For this review, take the finished solid that the model builds, in its own axes (mm). Face numbers are marked on the shaded views. A direction names the side the tool comes from. Coordinates: 2 decimals unless noted, no trailing zeros. Loops run counter-clockwise (first coordinate to the right, second up) from the corner with the lowest first, then second, coordinate; pieces in that order, holes last. Notation, with made-up numbers: (44.25, 62) - (54.25, 62) arc R29 cw to (54.25, 95) - close; hole circle Ø5 at (-20.5, 19.25). An arc over 180 degrees is marked (long way). Answer as a JSON object with one key per item and string values. Group by question number.
Item 1: We need section A-A (z = 11). Give the boundary of the cut face in (x, y).
Item 2: Tool access review of the marked faces 4 and 5: name each direction out of +Z, -Z, +X, -X, +Y, -Y from which nothing blocks a thin tool from reaching the whole face with its end or side.
Item 3: Mouldability with a two-part tool opening along X and no side actions: class the marked faces 1, 2 and 3 as released by +X, released by -X, zero draft, split by the parting line, or undercut.
Item 4: We need section C-C (z = 18). Give the boundary of the cut face in (x, y).
Item 5: To check wall thickness, follow line 1 (X direction, y = -19.1, z = 25); line 2 (Z direction, x = 7.5, y = -18); line 3 (Z direction, x = 8, y = -18.8). State the ranges of each line that lie inside material, in increasing order.
Item 6: We need section D-D (y = 3). Give the boundary of the cut face in (x, z).
Item 7: We need section B-B (x = 0). Give the boundary of the cut face in (y, z), then the cut area to 3 significant figures.
Item 8: Clearance check with flat-ended pins moving along their axes: pin 1 (10 mm diameter, centred on x = 3, y = -15, fed in from +Z); pin 2 (13 mm diameter, centred on x = 0, z = 18, fed in from +Y); pin 3 (2 mm diameter, centred on x = 2, y = 9, fed in from +Z). State where each tip first meets the part, or that it passes through.
from build123d import *

# Parameters (mm, degrees)
EXTRUDE_1_DEPTH          = 3
SKETCH_2_W               = 26.5
SKETCH_2_H               = 3
EXTRUDE_2_DEPTH          = 30
FILLET_1_R               = 3
FILLET_2_R               = 3
CUT_EXTRUDE_1_DEPTH      = 41.677082
CUT_EXTRUDE_1_DEPTH_BACK = 41.677082
SKETCH_3_R               = 4
CUT_EXTRUDE_2_DEPTH      = 41.677082
CUT_EXTRUDE_2_DEPTH_BACK = 41.677082
SKETCH_4_R               = 1.6
CUT_EXTRUDE_3_DEPTH      = 49.513529041
CUT_EXTRUDE_3_DEPTH_BACK = 49.513529041
SKETCH_5_R               = 5
CUT_EXTRUDE_4_DEPTH      = 49.513529041
CUT_EXTRUDE_4_DEPTH_BACK = 49.513529041
SKETCH_6_R               = 1.8


with BuildPart() as part:
    # 草图1 → 凸台-拉伸1 (new body)
    with BuildSketch(Plane.XY):
        with BuildLine():
            Line((13.25, 0), (13.25, -19.75))
            Line((13.25, -19.75), (-13.25, -19.75))
            Line((-13.25, -19.75), (-13.25, 0))
            ThreePointArc((-13.25, 0), (0, 13.25), (13.25, 0))
        make_face()
    extrude(amount=EXTRUDE_1_DEPTH)

    # 草图2 → 凸台-拉伸2 (add)
    with BuildSketch(Plane.XY.offset(3)):
        with Locations((0, -18.25)):
            Rectangle(SKETCH_2_W, SKETCH_2_H)
    extrude(amount=EXTRUDE_2_DEPTH)

    # 圆角1
    fillet_1_edges = [part.edges().sort_by_distance(p)[0] for p in [
        (0, -19.75, 0),
    ]]
    fillet(fillet_1_edges, radius=FILLET_1_R)

    # 圆角2
    fillet_2_edges = [part.edges().sort_by_distance(p)[0] for p in [
        (-13.25, -18.25, 33),
        (13.25, -18.25, 33),
    ]]
    fillet(fillet_2_edges, radius=FILLET_2_R)

    # 草图3 → 切除-拉伸1 (cut, two sides: drawn at the far end of the back side and taken through both)
    with BuildSketch(Plane(origin=(0, 0, 0), x_dir=(-1, 0, 0), z_dir=(0, 0, -1)).offset(-CUT_EXTRUDE_1_DEPTH_BACK)):
        with Locations(Location((0, 0, 0), (0, 0, 180))):
            Circle(SKETCH_3_R)
    extrude(amount=CUT_EXTRUDE_1_DEPTH + CUT_EXTRUDE_1_DEPTH_BACK, mode=Mode.SUBTRACT)

    # 草图4 → 切除-拉伸2 (cut, two sides: drawn at the far end of the back side and taken through both)
    with BuildSketch(Plane(origin=(0, 0, 0), x_dir=(-1, 0, 0), z_dir=(0, 0, -1)).offset(-CUT_EXTRUDE_2_DEPTH_BACK)):
        with Locations(Location((8.121035447, 0, 0), (0, 0, 180))):
            Circle(SKETCH_4_R)
        with Locations(Location((-7.851829852, 0, 0), (0, 0, 180))):
            Circle(SKETCH_4_R)
    extrude(amount=CUT_EXTRUDE_2_DEPTH + CUT_EXTRUDE_2_DEPTH_BACK, mode=Mode.SUBTRACT)

    # 草图5 → 切除-拉伸3 (cut, two sides: drawn at the far end of the back side and taken through both)
    with BuildSketch(Plane(origin=(0, -19.75, 0), x_dir=(-1, 0, 0), z_dir=(0, -1, 0)).offset(-CUT_EXTRUDE_3_DEPTH_BACK)):
        with Locations(Location((0, -18, 0), (0, 0, 90))):
            Circle(SKETCH_5_R)
    extrude(amount=CUT_EXTRUDE_3_DEPTH + CUT_EXTRUDE_3_DEPTH_BACK, mode=Mode.SUBTRACT)

    # 草图6 → 切除-拉伸4 (cut, two sides: drawn at the far end of the back side and taken through both)
    with BuildSketch(Plane(origin=(0, -19.75, 0), x_dir=(-1, 0, 0), z_dir=(0, -1, 0)).offset(-CUT_EXTRUDE_4_DEPTH_BACK)):
        with Locations(Location((-8, -11, 0), (0, 0, 90))):
            Circle(SKETCH_6_R)
        with Locations(Location((8, -11, 0), (0, 0, 90))):
            Circle(SKETCH_6_R)
        with Locations(Location((8, -25, 0), (0, 0, 90))):
            Circle(SKETCH_6_R)
        with Locations(Location((-8, -25, 0), (0, 0, 90))):
            Circle(SKETCH_6_R)
    extrude(amount=CUT_EXTRUDE_4_DEPTH + CUT_EXTRUDE_4_DEPTH_BACK, mode=Mode.SUBTRACT)


solid = part.part
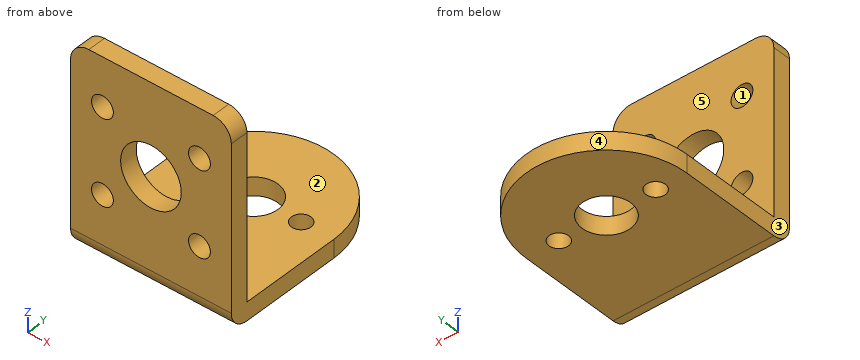
Check sheet entries:
{
 "1": {"outline": "(-13.25, -19.75) - (-9.8, -19.75) - (-9.8, -16.75) - (-13.25, -16.75) - close; (-6.2, -19.75) - (6.2, -19.75) - (6.2, -16.75) - (-6.2, -16.75) - close; (9.8, -19.75) - (13.25, -19.75) - (13.25, -16.75) - (9.8, -16.75) - close"},
 "2": {"face 4": "+Z, -Z, +Y", "face 5": "+Z, +X, -X, +Y"},
 "3": {"face 1": "undercut", "face 2": "zero draft", "face 3": "released by -X"},
 "4": {"outline": "(-13.25, -19.75) - (-5, -19.75) - (-5, -16.75) - (-13.25, -16.75) - close; (5, -19.75) - (13.25, -19.75) - (13.25, -16.75) - (5, -16.75) - close"},
 "5": {"line 1": "x = -13.25 to -9.8, -6.2 to 6.2, 9.8 to 13.25", "line 2": "z = 0.27 to 9.27, 12.73 to 23.27, 26.73 to 33", "line 3": "z = 0.81 to 9.2, 12.8 to 23.2, 26.8 to 33"},
 "6": {"outline": "(-12.91, 0) - (-2.65, 0) - (-2.65, 3) - (-12.91, 3) - close; (2.65, 0) - (12.91, 0) - (12.91, 3) - (2.65, 3) - close"},
 "7": {"outline": "(-19.75, 3) arc R3 ccw to (-16.75, 0) - (-4, 0) - (-4, 3) - (-16.75, 3) - (-16.75, 13) - (-19.75, 13) - close; (-19.75, 23) - (-16.75, 23) - (-16.75, 33) - (-19.75, 33) - close; (4, 0) - (13.25, 0) - (13.25, 3) - (4, 3) - close", "area": "133 mm2"},
 "8": {"pin 1": "stops at z = 33", "pin 2": "stops at y = -16.75", "pin 3": "stops at z = 3"}
}
